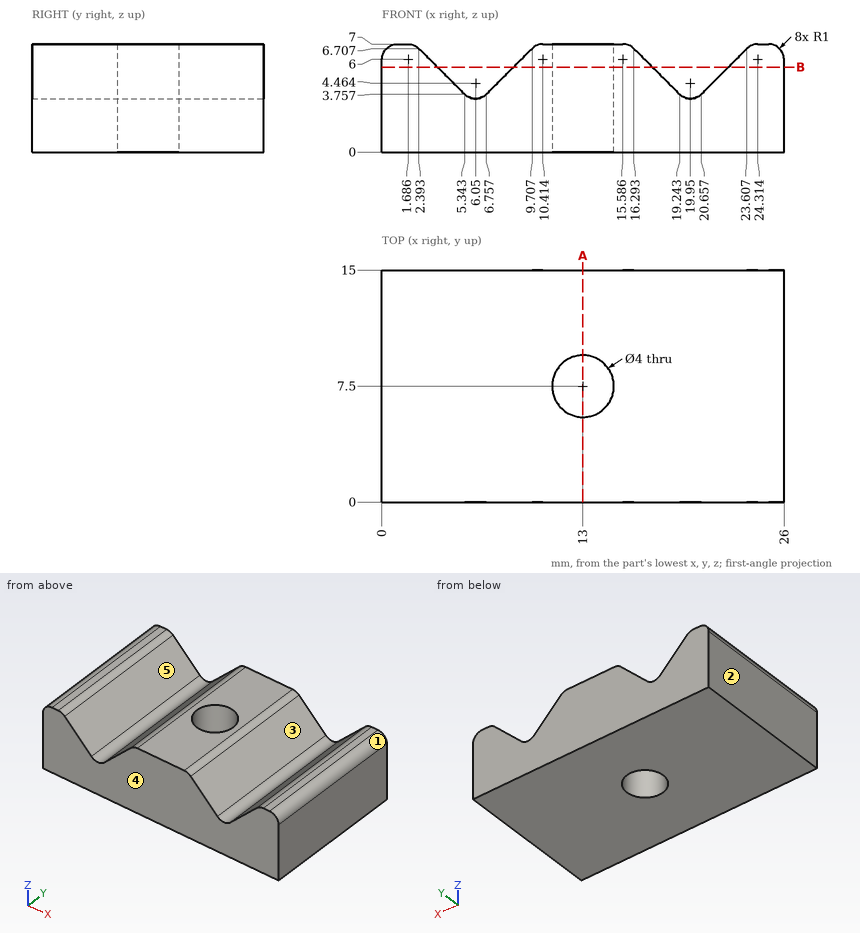
Design review of the part shown in the three views and the two pictorial views. Dimensions are in mm from the part's minimum x, y and z. A direction names the side the tool comes from. Coordinates: 2 decimals unless noted, no trailing zeros. Order: outer loops, then holes, each group sorted by start corner. A loop starts at its lowest first (then second) coordinate and runs counter-clockwise, first axis right, second up.
Item 1: For pin 1 Ø4 at (x, y) = (8, 7.5) entering from +Z, flat-tipped, find the tip position at first contact; note if it passes through.
Item 2: Take a section at A-A, the plane x = 13. Write out the cut boundary in (y, z).
Item 3: For the marked faces 4 and 5, list the 3-axis set-ups (+Z, -Z, +X, -X, +Y, -Y) from which the entire face can be reached by the end or side of a thin tool; tool diameter is ignored.
Item 4: The part is to be moulded in two halves that separate along X. For the marked faces 1, 2 and 3, say which applies: pulls with the +X half, pulls with the -X half, needs draft (parallel to the pull), parting line crosses it, or undercut.
Item 5: For line 1 (Y direction, x = 13, z = 2.75); line 2 (X direction, y = 14.75, z = 5); line 3 (X direction, y = 9, z = 4) (1 decimal), list the stretches that pass through material, from the lowest coordinate up.
Item 6: Take a section at B-B, the plane z = 5.5. Write out the cut boundary in (x, y).
The answers:
1. pin 1: stops at z = 6.91
2. outline: (0, 0) - (5.5, 0) - (5.5, 7) - (0, 7) - close; (9.5, 0) - (15, 0) - (15, 7) - (9.5, 7) - close
3. face 4: +Z, -Z, +X, -X, -Y
3. face 5: +Z, +Y, -Y
4. face 1: pulls with the +X half
4. face 2: pulls with the -X half
4. face 3: undercut
5. line 1: y = 0 to 5.5, 9.5 to 15
5. line 2: x = 0 to 4.1, 8 to 18, 21.9 to 26
5. line 3: x = 0 to 5.1, 7 to 11.7, 14.3 to 19, 20.9 to 26
6. outline: (0, 0) - (3.6, 0) - (3.6, 15) - (0, 15) - close; (8.5, 0) - (17.5, 0) - (17.5, 15) - (8.5, 15) - close; (22.4, 0) - (26, 0) - (26, 15) - (22.4, 15) - close; hole circle Ø4 at (13, 7.5)
